For this review, use the dimensioned drawing (mm, ordinates from the lowest corner) and the shaded views. Give positions to 0.01 mm unless a question says otherwise; leave off trailing zeros. Write each loop counter-clockwise with the first axis right and the second up, starting at its lowest first coordinate (ties: lowest second). Pieces come first, ordered by that corner, then holes. Notation, with made-up numbers: M 39.25,43.25 L 72.25,43.25 A18 cw 72.25,73.25 Z; hole C 56.5,78 d5. An arc over 180 degrees is marked long. One line per item, written item: value. Start each with the question number.
Item 1: Consider section A-A, the plane z = 1.5. Write out the cut boundary in (x, y), and give its area (3 significant figures).
Item 2: Consider section B-B, the plane x = 3. Write out the cut boundary in (y, z), and give its area (3 significant figures).
Item 3: To check wall thickness, follow probe 1 along Y at (x, z) = (3, 0.8); probe 2 along Z at (x, y) = (11.75, 7); probe 3 along X at (y, z) = (1.5, 0.7). State the ranges of each line that lie inside material, in increasing order.
Item 4: Mouldability with a two-part tool opening along Y and no side actions: class the marked faces 1, 2 and 3 as released by +Y, released by -Y, zero draft, split by the parting line, or undercut.
Item 5: Consider section C-C, the plane x = 5.25. Write out the cut boundary in (y, z).
Item 6: Clearance check with flat-ended pins moving along their axes: pin 1 Ø0.8 at (y, z) = (19.5, 2.5) entering from -X; pin 2 Ø1.5 at (x, y) = (12.5, 22) entering from -Z; pin 3 Ø0.6 at (y, z) = (11, 2.5) entering from +X. State where each tip first meets the part, or that it passes through.
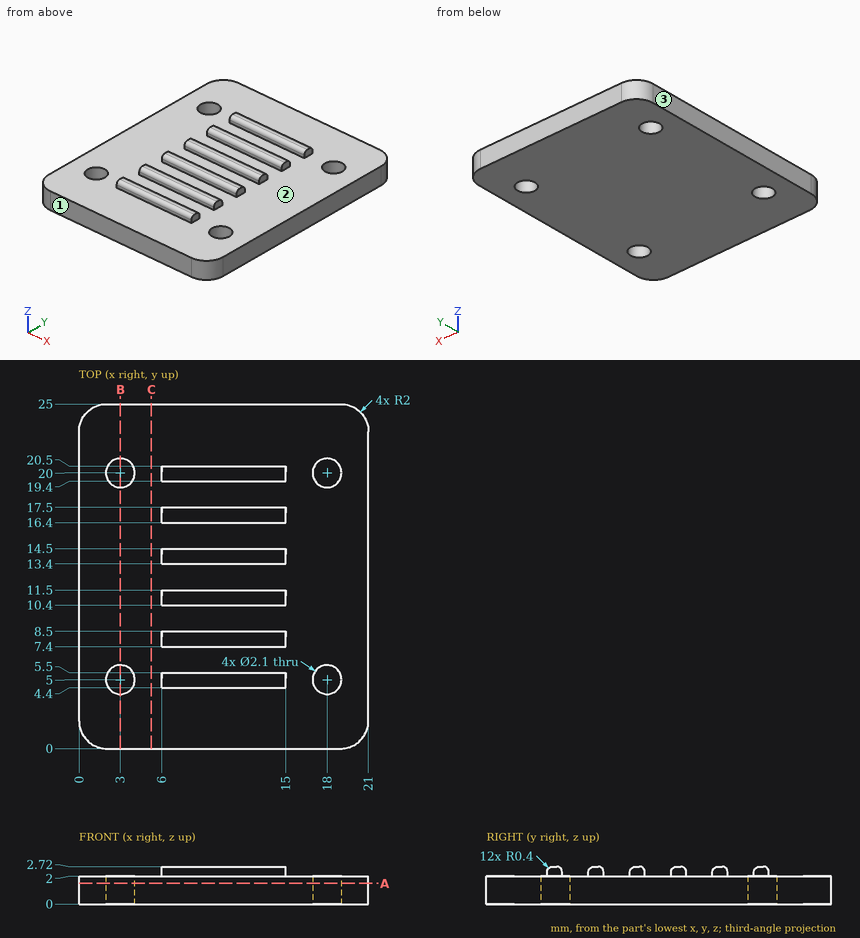
Model answer:
1. outline: M 0,2 A2 ccw 2,0 L 19,0 A2 ccw 21,2 L 21,23 A2 ccw 19,25 L 2,25 A2 ccw 0,23 Z; hole C 3,5 d2.1; hole C 3,20 d2.1; hole C 18,5 d2.1; hole C 18,20 d2.1
1. area: 508 mm2
2. outline: M 0,0 L 3.95,0 L 3.95,2 L 0,2 Z; M 6.05,0 L 18.95,0 L 18.95,2 L 6.05,2 Z; M 21.05,0 L 25,0 L 25,2 L 21.05,2 Z
2. area: 41.6 mm2
3. probe 1: y = 0 to 3.95, 6.05 to 18.95, 21.05 to 25
3. probe 2: z = 0 to 2
3. probe 3: x = 0.06 to 20.94
4. face 1: released by -Y
4. face 2: undercut
4. face 3: zero draft
5. outline: M 0,0 L 25,0 L 25,2 L 0,2 Z
6. pin 1: stops at x = 6
6. pin 2: stops at z = 0
6. pin 3: stops at x = 15
